Autodesk Inventor part; units mm, degrees
ref_plane "YZ Plane" through (0, 0, 0) normal (1, 0, 0) x (0, 1, 0)
ref_plane "XZ Plane" through (0, 0, 0) normal (0, 1, 0) x (-1, 0, 0)
ref_plane "XY Plane" through (0, 0, 0) normal (0, 0, 1) x (1, 0, 0)
sketch "Skizze1" plane through (0, 0, 0) normal (0, 1, 0) x (-1, 0, 0)
  line L0 (0, 0) -> (-25.4, 0)
  line L1 (-25.4, 0) -> (-25.4, 75.5)
  line L2 (-25.4, 75.5) -> (0, 75.5)
  line L3 (0, 75.5) -> (0, 0)
  dimension "d0" = 25.4
  dimension "d1" = 75.5
extrude "Extrusion1" add sketch "Skizze1" along normal blind 1
sketch "Skizze2" plane through (0, 1, 0) normal (0, 1, 0) x (1, 0, 0)
  line L0 (0, -75.5) -> (25.4, -75.5)
  line L1 (25.4, -75.5) -> (25.4, 0)
  line L2 (25.4, 0) -> (0, 0)
  line L3 (0, 0) -> (0, -75.5)
  line L4 (7, -60) -> (18.4, -60)
  line L5 (18.4, -60) -> (18.4, -15.5)
  line L6 (18.4, -15.5) -> (7, -15.5)
  line L7 (7, -15.5) -> (7, -60)
  dimension "d4" = 7
  dimension "d5" = 7
  dimension "d6" = 15.5
  dimension "d7" = 15.5
extrude "Extrusion2" add sketch "Skizze2" along normal blind 7.5 contours L7 L6 L5 L4
sketch "Skizze3" plane through (0, 8.5, 0) normal (0, 1, 0) x (1, 0, 0)
  line L0 (18.4, -60) -> (18.4, -15.5)
  line L1 (18.4, -15.5) -> (7, -15.5)
  line L2 (7, -15.5) -> (7, -60)
  line L3 (7, -60) -> (18.4, -60)
  circle A0 centre (12.7, -53) radius 1.7919
  circle A1 centre (12.7, -22.5) radius 1.7997
  point P0 (0, 0)
  dimension "d10" = 7
  dimension "d11" = 7
extrude "Extrusion3" cut sketch "Skizze3" against normal up to surface (7.5 mm away) contours A0 | A1
ref_plane "Arbeitsebene1" through (12.7, 0, 75.5) normal (1, 0, 0) x (0, 0, -1)
sketch "Skizze5" plane through (12.7, 1, 60) normal (1, 0, 0) x (0, 0, -1)
  line L0 (8.3796, 0.5) -> (36.1482, 0.5)
  line L1 (-15.5, 0) -> (60, 0)
  line L2 (8.7919, 7.5) -> (8.7919, 0)
  line L3 (8.7919, 1.6191) -> (12.5, 1.6191)
  line L4 (12.5, 1.6191) -> (22, 0.7063)
  line L5 (22, 0.7063) -> (22, 0.5)
  line L6 (36.1103, 0.5) -> (8.3796, 0.5)
  line L7 (0, 0) -> (0, 7.5)
  line L8 (-15.5, -1) -> (-15.5, 0)
  line L9 (60, -1) -> (60, 0)
  line L10 (35.7003, 7.5) -> (35.7003, 0)
  line L11 (44.5, 0) -> (0, 0)
  line L12 (35.7003, 0.5) -> (8.7919, 0.5)
  line L13 (8.7919, 0.5) -> (8.7919, 0)
  line L14 (8.7919, 0) -> (35.7003, 0)
  line L15 (35.7003, 0) -> (35.7003, 0.5)
  line L16 (8.7919, 1.6191) -> (8.7919, 0.5)
  point P0 (35.7003, 0.5)
  point P1 (22, 0.5)
  dimension "d17" = 28
  dimension "d18" = 38
extrude "Extrusion5" cut sketch "Skizze5" along normal mid plane 2
sketch "Skizze6" plane through (0, 0, 0) normal (0, -1, 0) x (1, 0, 0)
  line L0 (13.7, 47.5) -> (11.7, 47.5)
  line L1 (11.7, 38) -> (13.7, 38)
  circle A0 centre (12.7, 40.1939) radius 1.0539
  point P0 (0, 0)
extrude "Extrusion6" cut sketch "Skizze6" against normal blind 0.1
equation "\"d12\" = d11"
properties part number "00_chip"
Model file for the job. Use its own axes, mm. A direction names the side the tool comes from. Give positions to 0.01 mm unless a question says otherwise; leave off trailing zeros. Write each loop counter-clockwise with the first axis right and the second up, starting at its lowest first coordinate (ties: lowest second). Pieces come first, ordered by that corner, then holes. Notation, with made-up numbers: M 7.5,12.25 L 55.5,12.25 A35 cw 55.5,46.25 Z; hole C -31,21 d11. An arc over 180 degrees is marked long. Use a Markdown table: item, result.
1) Cut at D-D (z = 27.5). List the corners of the cut face in (x, y).
Responses:
| item | result |
|---|---|
| outline | M 0,0 L 25.4,0 L 25.4,1 L 18.4,1 L 18.4,8.5 L 7,8.5 L 7,1 L 0,1 Z; hole M 11.7,1 L 13.7,1 L 13.7,1.5 L 11.7,1.5 Z |
2) Drill centre lines: line 1 (Z direction, x = 12.7, y = 4.75); line 2 (Y direction, x = 5.5, z = 8.5); line 3 (Z direction, x = 8.5, y = 3.25). Where is each one in solid material? Low to high. Write a range as from..to.
Responses:
| item | result |
|---|---|
| line 1 | z = 15.5..20.7, 24.3..51.21, 54.79..60 |
| line 2 | y = 0..1 |
| line 3 | z = 15.5..60 |
3) Tool access for faces 1 (the flat face through (13, 0.1, 40)), 2 (the flat face through (11.7, 1.6, 40.9)), 3 (the flat face through (7, 5, 37)), 4 (the flat face through (13, 5, 60)), 5 (the cylindrical face through (12.466, 4.802, 20.716)): list every direction of +Z, -Z, +X, -X, +Y, -Y with a clear straight run to the whole face (end or side of a thin tool).
Responses:
| item | result |
|---|---|
| face 1 | -Y |
| face 2 | none |
| face 3 | +Z, -Z, -X, +Y |
| face 4 | +Z, +X, -X, +Y |
| face 5 | +Y |
4) Pin check, flat tips, straight feed: pin 1 (0.6 mm diameter, centred on x = 13, z = 32, fed in from -Y); pin 2 (1 mm diameter, centred on y = 2, z = 60, fed in from -X); pin 3 (1.1 mm diameter, centred on x = 12.5, z = 40.5, fed in from -Y); pin 4 (1.5 mm diameter, centred on y = 6, z = 20, fed in from +X). Stop position of each tip, or through.
Responses:
| item | result |
|---|---|
| pin 1 | stops at y = 0 |
| pin 2 | stops at x = 7 |
| pin 3 | stops at y = 0.1 |
| pin 4 | stops at x = 18.4 |
5) Cut at C-C (x = 17.75). List the corners of the cut face in (y, z), and give its area (3 significant figures).
Responses:
| item | result |
|---|---|
| outline | M 0,0 L 1,0 L 1,15.5 L 8.5,15.5 L 8.5,60 L 1,60 L 1,75.5 L 0,75.5 Z |
| area | 409 mm2 |
6) Cut at A-A (y = 7.5). List the corners of the cut face in (x, z), and give its area (3 significant figures).
Responses:
| item | result |
|---|---|
| outline | M 7,15.5 L 18.4,15.5 L 18.4,60 L 7,60 Z; hole C 12.7,22.5 d3.6; hole C 12.7,53 d3.58 |
| area | 487 mm2 |
7) Cut at B-B (z = 53). List the corners of the cut face in (x, y).
Responses:
| item | result |
|---|---|
| outline | M 0,0 L 25.4,0 L 25.4,1 L 18.4,1 L 18.4,8.5 L 14.49,8.5 L 14.49,1 L 10.91,1 L 10.91,8.5 L 7,8.5 L 7,1 L 0,1 Z |
8) Pull direction Y, two halves, no side cores. Call faces 6 (the flat face through (13, 5, 15.5)), 7 (the flat face through (13, 1, 38)), 8 (the flat face through (13, 8.5, 37)), 9 (the flat face through (13, 0, 38)): +Y half, -Y half, draft (parallel to the pull), parting line (faces both ways), or undercut.
Responses:
| item | result |
|---|---|
| face 6 | draft |
| face 7 | undercut |
| face 8 | +Y half |
| face 9 | -Y half |
